from build123d import *

# Parameters (mm, degrees)
F0_R     = 17.5
F1_DEPTH = 2.5
F2_R     = 17.5
F3_DEPTH = 50
F3_TAPER = 15
F4_R     = 3.6137849114
F5_DEPTH = 60


with BuildPart() as f1:
    # F0 (on Top) → F1 (new body)
    with BuildSketch(Plane.XY):
        with BuildLine():
            Line((0, 38.8068709316), (-35.2930977718, 38.8068709316))
            ThreePointArc((-35.2930977718, 38.8068709316), (-38.8286316778, 37.3424048375), (-40.2930977718, 33.8068709316))
            Line((-40.2930977718, 33.8068709316), (-40.2930977718, 0))
            ThreePointArc((-40.2930977718, 0), (-38.8286316778, -3.5355339059), (-35.2930977718, -5))
            Line((-35.2930977718, -5), (0, -5))
            ThreePointArc((0, -5), (3.5355339059, -3.5355339059), (5, 0))
            Line((5, 0), (5, 33.8068709316))
            ThreePointArc((5, 33.8068709316), (3.5355339059, 37.3424048375), (0, 38.8068709316))
        make_face()
        with Locations((-17.6465488859, 16.9034354658)):
            Circle(F0_R, mode=Mode.SUBTRACT)
        with Locations((-17.6465488859, 16.9034354658)):
            Circle(F0_R)
    extrude(amount=F1_DEPTH)

    # F2 (on face) → F3 (join)
    with BuildSketch(Plane.XY.offset(2.5)):
        with Locations((-17.6465488859, 16.9034354658)):
            Circle(F2_R)
    extrude(amount=F3_DEPTH, taper=F3_TAPER)

    # F4 (on Right) → F5 (cut)
    with BuildSketch(Plane.YZ):
        with Locations((17.7631601691, 42.927633971)):
            Circle(F4_R)
    extrude(amount=-F5_DEPTH, mode=Mode.SUBTRACT)


solid = f1.part
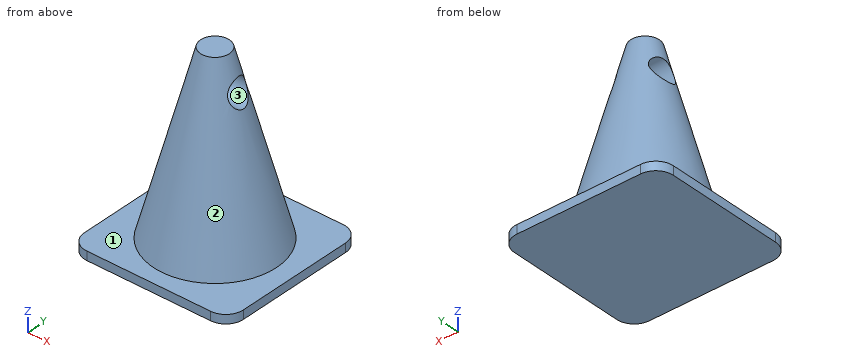
Geometry check sheet. Reference: the model listing, model coordinates, mm. Face numbers are marked on the shaded views. Give positions to 0.01 mm unless a question says otherwise; leave off trailing zeros. Write each loop counter-clockwise with the first axis right and the second up, starting at its lowest first coordinate (ties: lowest second). Pieces come first, ordered by that corner, then holes. Notation, with made-up numbers: M 47,38.25 L 52,38.25 A26 cw 52,68.25 Z; hole C -3,25.25 d10. An arc over 180 degrees is marked long. One line per question, with ' | ' between items.
1. Cross-section at B-B (x = -36.5). Enter the section's corners in (y, z).
Ans:
outline: M -4.85,0 L 38.66,0 L 38.66,2.5 L -4.85,2.5 Z
2. Cross-section at A-A (z = 9). Enter the section's corners in (x, y).
Ans:
outline: C -17.65,16.9 d31.52
3. Cross-section at C-C (z = 36). Enter the section's corners in (x, y), plus the area to 3 significant figures.
Ans:
outline: C -17.65,16.9 d17.05 | area: 228 mm2
4. Scan lines: line 1 along Z through (x, y) = (3, 6.5); line 2 along Y through (x, z) = (-17, 44); line 3 along Z through (x, y) = (-16, 14.5). Record each from-to range of solid material in increasing order. Write a range as from..to.
Ans:
line 1: 0..2.5 | line 2: 10.56..14.31, 21.21..23.25 | line 3: 0..41.37, 44.48..52.5
5. Gauge pin test, flat ends, axial feed: pin 1 (9.5 mm diameter, centred on y = 17.76, z = 42.93, fed in from -X); pin 2 (5 mm diameter, centred on x = -35.5, y = 5.5, fed in from +Z); pin 3 (1 mm diameter, centred on x = -20.5, z = 6, fed in from -Y). Record the tip position at first contact, or that the pin passes through.
Ans:
pin 1: x = -25.57 | pin 2: z = 2.5 | pin 3: y = 0.43
6. Mould release check, pull along Y, two halves, no side actions. Record for the marked faces 1, 2 and 3: released by +Y, released by -Y, zero draft, split by the parting line, or undercut.
Ans:
face 1: zero draft | face 2: split by the parting line | face 3: undercut
